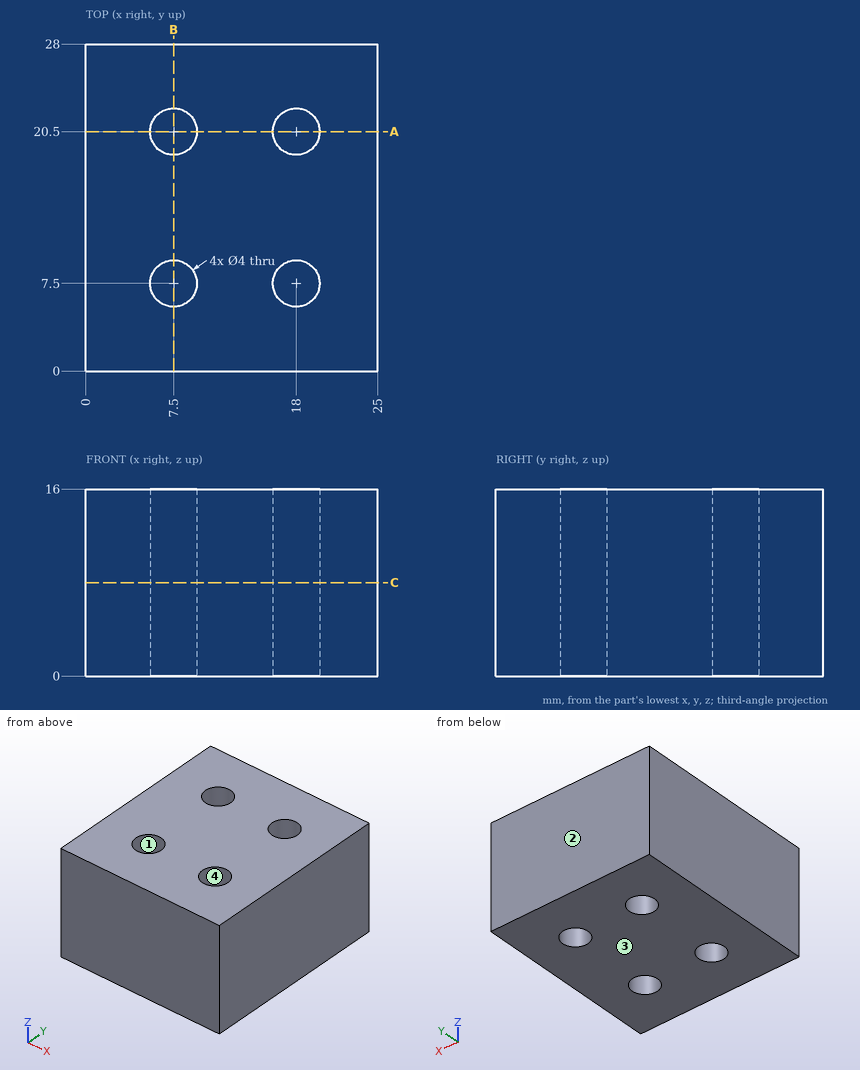
Could you check a few things on this drawing? It's one solid part, dimensions in mm from its lowest x, y, z. Coordinates: 2 decimals unless noted, no trailing zeros. Order: outer loops, then holes, each group sorted by start corner. A loop starts at its lowest first (then second) coordinate and runs counter-clockwise, first axis right, second up. Notation, with made-up numbers: M 32.5,69 L 66.5,69 A24 ccw 66.5,99 Z; hole C 64,-22 d8. An arc over 180 degrees is marked long. Use one line per item in the form item = value. Start each with the question number.
1. Please list where these lines run through material, in increasing order: line 1 (Y direction, x = 18, z = 4); line 2 (Y direction, x = 8, z = 7); line 3 (X direction, y = 20.75, z = 4.5).
2. For pin 1 (2.5 mm diameter, centred on x = 18, y = 7.5, fed in from +Z), with a flat end and sliding along its axis, tell me the tip position at first contact or that it passes through.
3. Suppose I cut it at A-A on y = 20.5. Write out the boundary of the cut face in (x, z), then the cut area to 3 significant figures.
4. We'd pull the mould along Y, two halves only. Please class the marked faces 1, 2, 3 and 4: +Y half, -Y half, draft (parallel to the pull), parting line (faces both ways), or undercut.
5. Suppose I cut it at C-C on z = 8. Write out the boundary of the cut face in (x, y).
6. Suppose I cut it at B-B on x = 7.5. Write out the boundary of the cut face in (y, z).
Geometry says:
q1.line_1 = 0 to 5.5, 9.5 to 18.5, 22.5 to 28
q1.line_2 = 0 to 5.56, 9.44 to 18.56, 22.44 to 28
q1.line_3 = 0 to 5.52, 9.48 to 16.02, 19.98 to 25
q2.pin_1 = through
q3.outline = M 0,0 L 5.5,0 L 5.5,16 L 0,16 Z; M 9.5,0 L 16,0 L 16,16 L 9.5,16 Z; M 20,0 L 25,0 L 25,16 L 20,16 Z
q3.area = 272 mm^2
q4.face_1 = undercut
q4.face_2 = +Y half
q4.face_3 = draft
q4.face_4 = undercut
q5.outline = M 0,0 L 25,0 L 25,28 L 0,28 Z; hole C 7.5,7.5 d4; hole C 7.5,20.5 d4; hole C 18,7.5 d4; hole C 18,20.5 d4
q6.outline = M 0,0 L 5.5,0 L 5.5,16 L 0,16 Z; M 9.5,0 L 18.5,0 L 18.5,16 L 9.5,16 Z; M 22.5,0 L 28,0 L 28,16 L 22.5,16 Z
